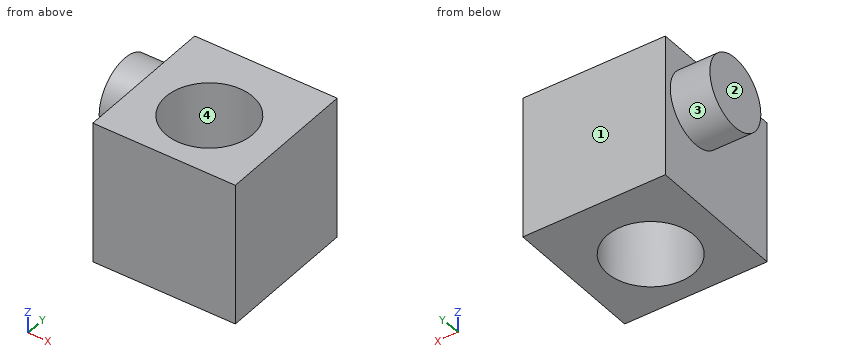
```python
from build123d import *

# Parameters (mm, degrees)
F0_W     = 90
F0_H     = 90
F1_DEPTH = 90
F2_R     = 27.5
F3_DEPTH = 90
F4_R     = 22.5
F5_DEPTH = 25


with BuildPart() as f1:
    # F0 (on Front) → F1 (new body)
    with BuildSketch(Plane.XZ):
        with Locations((2.812499, 10.546107)):
            Rectangle(F0_W, F0_H)
    extrude(amount=F1_DEPTH)

    # F2 (on face) → F3 (cut, through all)
    with BuildSketch(Plane.XY.offset(55.546107)):
        with Locations((2.812499, -50)):
            Circle(F2_R)
    extrude(amount=-F3_DEPTH, mode=Mode.SUBTRACT)

    # F4 (on face) → F5 (join)
    with BuildSketch(Plane(origin=(-42.187501, 0, 0), x_dir=(0, -1, 0), z_dir=(-1, 0, 0))):
        with Locations((26.878221, 24.340734)):
            Circle(F4_R)
    extrude(amount=F5_DEPTH)


solid = f1.part
```
Can you work these out from the model? Positions are in its coordinate system, mm. Face numbers are marked on the shaded views. Coordinates: 2 decimals unless noted, no trailing zeros. Order: outer loops, then holes, each group sorted by start corner. A loop starts at its lowest first (then second) coordinate and runs counter-clockwise, first axis right, second up. Notation, with made-up numbers: (11, 67) - (65, 67) arc R14 ccw to (65, 81) - close; hole circle Ø8 at (21, 18). An arc over 180 degrees is marked (long way). Answer in a Markdown table with one row per item.
1. If we mould it in two halves opening along Y, with no side actions, what happens to the marked faces 1, 2, 3 and 4? For each: pulls with the +Y half, pulls with the -Y half, needs draft (parallel to the pull), parting line crosses it, or undercut.
Reply:
| item | result |
|---|---|
| face 1 | pulls with the +Y half |
| face 2 | needs draft |
| face 3 | parting line crosses it |
| face 4 | undercut |
2. If I drill on line 1 along Y through (x, z) = (25.5, 33); line 2 along Y through (x, z) = (23, 43); line 3 along X through (y, z) = (-16, 45), over which ranges is the centre line in solid material (lowest first)?
Reply:
| item | result |
|---|---|
| line 1 | y = -90 to -65.54, -34.46 to 0 |
| line 2 | y = -90 to -68.67, -31.33 to 0 |
| line 3 | x = -42.19 to 47.81 |
3. Suppose I cut it at C-C (x = -14). Please give me the cut outline in (y, z).
Reply:
| item | result |
|---|---|
| outline | (-90, -34.45) - (-71.76, -34.45) - (-71.76, 55.55) - (-90, 55.55) - close; (-28.24, -34.45) - (0, -34.45) - (0, 55.55) - (-28.24, 55.55) - close |
4. Suppose I cut it at D-D (y = -12.5). Please give me the cut outline in (x, z), and give its area (3 significant figures).
Reply:
| item | result |
|---|---|
| outline | (-67.19, 7.03) - (-42.19, 7.03) - (-42.19, -34.45) - (47.81, -34.45) - (47.81, 55.55) - (-42.19, 55.55) - (-42.19, 41.65) - (-67.19, 41.65) - close |
| area | 8,970 mm^2 |
5. For pin 1 (12 mm diameter, centred on x = -54, y = -39, fed in from -Z), with a flat end and sliding along its axis, tell me the tip position at first contact or that it passes through.
Reply:
| item | result |
|---|---|
| pin 1 | stops at z = 2.69 |
6. Suppose I cut it at A-A (z = -0.5). Please give me the cut outline in (x, y).
Reply:
| item | result |
|---|---|
| outline | (-42.19, -90) - (47.81, -90) - (47.81, 0) - (-42.19, 0) - close; hole circle Ø55 at (2.81, -50) |
7. Suppose I cut it at B-B (y = -34). Please give me the cut outline in (x, z), and give its area (3 significant figures).
Reply:
| item | result |
|---|---|
| outline | (-67.19, 3) - (-42.19, 3) - (-42.19, -34.45) - (-19.55, -34.45) - (-19.55, 55.55) - (-42.19, 55.55) - (-42.19, 45.68) - (-67.19, 45.68) - close; (25.18, -34.45) - (47.81, -34.45) - (47.81, 55.55) - (25.18, 55.55) - close |
| area | 5,140 mm^2 |
